from build123d import *

# Parameters (mm, degrees)
BOSS_EXTRUDE3_DEPTH = 2
SKETCH7_R           = 1
SKETCH7_W           = 2.5
SKETCH7_H           = 2.5
BOSS_EXTRUDE5_DEPTH = 3


with BuildPart() as part:
    # Sketch2 → Boss-Extrude3 (new body)
    with BuildSketch(Plane.XY):
        Polygon((62.078732257, 67), (7.070378023, 67), (2.153513577, 62.087886246), (2.153513577, 6.916864445), (7.070378023, 2), (62.078732257, 2), (67.153513577, 7.083274694), (67.153513577, 61.921636784), align=None)
        with BuildLine():
            ThreePointArc((12.561398281, 29.386897281), (12.405099811, 29.087669445), (12.28230409, 28.773205265))
            ThreePointArc((12.28230409, 28.773205265), (9.332354964, 25.48092154), (6.384978263, 28.775508397))
            ThreePointArc((6.384978263, 28.775508397), (6.272687262, 29.080787813), (6.128559615, 29.372390302))
            ThreePointArc((6.128559615, 29.372390302), (9.319946418, 40.479834047), (12.561398281, 29.386897281))
        make_face(mode=Mode.SUBTRACT)
        with BuildLine():
            Line((7.315683042, 44.45), (3.053513577, 44.45))
            Line((3.053513577, 44.45), (3.053513577, 49.55))
            Line((3.053513577, 49.55), (15.603513577, 49.55))
            Line((15.603513577, 49.55), (15.603513577, 44.45))
            Line((15.603513577, 44.45), (11.175073004, 44.45))
            ThreePointArc((11.175073004, 44.45), (9.245378023, 45.49849), (7.315683042, 44.45))
        make_face(mode=Mode.SUBTRACT)
    extrude(amount=BOSS_EXTRUDE3_DEPTH)

    # Sketch7 → Boss-Extrude5 (add)
    with BuildSketch(Plane.XY.offset(2)):
        with BuildLine():
            Line((15.753513577, 14.57), (11.264187035, 14.57))
            ThreePointArc((11.264187035, 14.57), (9.333513577, 15.62), (7.40284012, 14.57))
            Line((7.40284012, 14.57), (2.153513577, 14.57))
            Line((2.153513577, 14.57), (2.153513577, 12.07))
            Line((2.153513577, 12.07), (7.033513577, 12.07))
            Line((7.033513577, 12.07), (7.40284012, 12.07))
            ThreePointArc((7.40284012, 12.07), (9.333513577, 11.02), (11.264187035, 12.07))
            Line((11.264187035, 12.07), (11.633513577, 12.07))
            Line((11.633513577, 12.07), (15.753513577, 12.07))
            Line((15.753513577, 12.07), (15.753513577, 14.57))
        make_face()
        with Locations((9.333513577, 13.32)):
            Circle(SKETCH7_R, mode=Mode.SUBTRACT)
        with BuildLine():
            Line((11.633513577, 9.547776159), (11.633513577, 12.07))
            Line((11.633513577, 12.07), (11.264187035, 12.07))
            ThreePointArc((11.264187035, 12.07), (9.333513577, 11.02), (7.40284012, 12.07))
            Line((7.40284012, 12.07), (7.033513577, 12.07))
            Line((7.033513577, 12.07), (7.033513577, 9.547776159))
            Line((7.033513577, 9.547776159), (11.633513577, 9.547776159))
        make_face()
        with Locations((17.003513577, 13.32)):
            Rectangle(SKETCH7_W, SKETCH7_H)
        with BuildLine():
            Line((15.753513577, 16.534568208), (15.753513577, 14.57))
            Line((15.753513577, 14.57), (18.253513577, 14.57))
            Line((18.253513577, 14.57), (18.253513577, 16.534568208))
            Line((18.253513577, 16.534568208), (18.253513577, 44.45))
            Line((18.253513577, 44.45), (15.753513577, 44.45))
            Line((15.753513577, 44.45), (15.753513577, 44.44849))
            Line((15.753513577, 44.44849), (11.17605148, 44.44849))
            ThreePointArc((11.17605148, 44.44849), (11.17556239, 44.449245096), (11.175073004, 44.45))
            ThreePointArc((11.175073004, 44.45), (10.343450652, 45.219439406), (9.245378023, 45.49849))
            ThreePointArc((9.245378023, 45.49849), (8.147305393, 45.219439406), (7.315683042, 44.45))
            ThreePointArc((7.315683042, 44.45), (7.315193656, 44.449245096), (7.314704565, 44.44849))
            Line((7.314704565, 44.44849), (2.153513577, 44.44849))
            Line((2.153513577, 44.44849), (2.153513577, 41.94849))
            Line((2.153513577, 41.94849), (7.314704565, 41.94849))
            ThreePointArc((7.314704565, 41.94849), (9.245378023, 40.89849), (11.17605148, 41.94849))
            Line((11.17605148, 41.94849), (15.753513577, 41.94849))
            Line((15.753513577, 41.94849), (15.753513577, 16.534568208))
        make_face()
        with Locations((9.245378023, 43.19849)):
            Circle(SKETCH7_R, mode=Mode.SUBTRACT)
    extrude(amount=BOSS_EXTRUDE5_DEPTH)


solid = part.part
Build history of the part. All positions in model axes, mm. A direction names the side the tool comes from. Give positions to 0.01 mm unless a question says otherwise; leave off trailing zeros. Order: outer loops, then holes, each group sorted by start corner. A loop starts at its lowest first (then second) coordinate and runs counter-clockwise, first axis right, second up. Notation, with made-up numbers: M -38.75,36.25 L -9.75,36.25 A35 ccw -9.75,69.25 Z; hole C 22.5,77.5 d4. An arc over 180 degrees is marked long. Use one line per item in the form item = value.
Q1. Slice it at C-C, the plane y = 13.32. Write the cut outline in (x, z).
Conclusion:
outline = M 2.15,0 L 67.15,0 L 67.15,2 L 18.25,2 L 18.25,5 L 10.33,5 L 10.33,2 L 8.33,2 L 8.33,5 L 2.15,5 Z
Q2. Wall check: probe 1 along Z at (x, y) = (64, 8); probe 2 along X at (y, z) = (19, 3.85); probe 3 along X at (y, z) = (12.5, 2.6). Give the ranges that are in metal, low to high.
Conclusion:
probe_1 = 0 to 2
probe_2 = 15.75 to 18.25
probe_3 = 2.15 to 8.76, 9.91 to 18.25
Q3. Which spindle directions (+Z, -Z, +X, -X, +Y, -Y) get a long thin tool onto all of the face, cutting with end or side? Do faces 4 (the flat face through (13, 41.948, 3)), 5 (the flat face through (9, 49.55, 1)), 6 (the flat face through (5, 14.57, 3)), 7 (the flat face through (17, 44.45, 3)), 8 (the flat face through (9, 9.548, 3)). Say none if no direction does.
Conclusion:
face_4 = +Z
face_5 = +Z, -Z
face_6 = +Z, -X
face_7 = +Z, +X, +Y
face_8 = +Z, +X, -X, -Y
Q4. Pull direction X, two halves, no side cores. Call faces 1 (the flat face through (5, 44.448, 3)), 2 (the flat face through (7.034, 11, 3)), 3 (the cylindrical face through (9.37, 15.62, 3.48)): released by +X, released by -X, zero draft, split by the parting line, or undercut.
Conclusion:
face_1 = zero draft
face_2 = released by -X
face_3 = undercut
Q5. Slice it at A-A, the plane y = 48.5. Write the cut outline in (x, z).
Conclusion:
outline = M 2.15,0 L 3.05,0 L 3.05,2 L 2.15,2 Z; M 15.6,0 L 67.15,0 L 67.15,2 L 15.6,2 Z
Q6. Slice it at B-B, the plane z = 1.1. Write the cut outline in (x, y).
Conclusion:
outline = M 2.15,6.92 L 7.07,2 L 62.08,2 L 67.15,7.08 L 67.15,61.92 L 62.08,67 L 7.07,67 L 2.15,62.09 Z; hole M 3.05,44.45 L 7.32,44.45 A2.3 cw 11.18,44.45 L 15.6,44.45 L 15.6,49.55 L 3.05,49.55 Z; hole M 6.13,29.37 A3.05 cw 6.38,28.78 A2.97 ccw long 12.28,28.77 A3.1 cw 12.56,29.39 A6.02 ccw long Z
Q7. Slice it at D-D, the plane x = 49. Write the cut outline in (y, z).
Conclusion:
outline = M 2,0 L 67,0 L 67,2 L 2,2 Z
Q8. Pin check, flat tips, straight feed: P1, Ø3, axis at x = 53.5, y = 58.5, coming from the +Z side; P2, Ø2.5, axis at x = 13, z = 3.5, coming from the +Y side; P3, Ø2, axis at x = 16.5, z = 4, coming from the +Y side. Stop position of each tip, or through.
Conclusion:
P1 = 2
P2 = 44.45
P3 = 44.45
